Geometry: final body of the model. Coordinates: model frame, mm. A direction names the side the tool comes from. Round coordinates to 2 decimals unless told otherwise and drop trailing zeros. Loops run counter-clockwise (first coordinate to the right, second up) from the corner with the lowest first, then second, coordinate; pieces in that order, holes last. Notation, with made-up numbers: M -16.75,45.25 L 10.25,45.25 A24 cw 10.25,84.25 Z; hole C 10,21.25 d6. An arc over 180 degrees is marked long. Answer as a JSON object with one key per item and string values.
from build123d import *

# Parameters (mm, degrees)
SKETCH2_W            = 91
SKETCH2_H            = 67
BOSS_EXTRUDE10_DEPTH = 55.68
CUT_EXTRUDE13_DEPTH  = 99
CUT_EXTRUDE14_DEPTH  = 99
SKETCH28_W           = 87
SKETCH28_H           = 97.65285099
CUT_EXTRUDE16_DEPTH  = 31
SKETCH29_W           = 91
SKETCH29_H           = 35
BOSS_EXTRUDE12_DEPTH = 34.25
SKETCH30_W           = 87
SKETCH30_H           = 34.25
CUT_EXTRUDE18_DEPTH  = 32.44
SKETCH31_W           = 34.25
SKETCH31_H           = 2.550055223
BOSS_EXTRUDE13_DEPTH = 13.42
SKETCH32_W           = 34.25
SKETCH32_H           = 2.55894211
BOSS_EXTRUDE14_DEPTH = 13.42
CUT_EXTRUDE19_DEPTH  = 13.42
CUT_EXTRUDE20_DEPTH  = 13.42
SKETCH35_W           = 91
SKETCH35_H           = 35
BOSS_EXTRUDE15_DEPTH = 3
CUT_EXTRUDE21_DEPTH  = 99
SKETCH38_W           = 91
SKETCH38_H           = 34.25
BOSS_EXTRUDE16_DEPTH = 7.58
SKETCH40_W           = 87
SKETCH40_H           = 31.930310383
CUT_EXTRUDE23_DEPTH  = 7.13


with BuildPart() as part:
    # Sketch2 → Boss-Extrude10 (new body)
    with BuildSketch(Plane(origin=(0, 0, 0), x_dir=(1, 0, 0), z_dir=(0, 1, 0))):
        with Locations((45.5, 33.5)):
            Rectangle(SKETCH2_W, SKETCH2_H)
    extrude(amount=BOSS_EXTRUDE10_DEPTH)

    # Sketch24 → Cut-Extrude13 (cut)
    with BuildSketch(Plane.ZY):
        Polygon((-67, 0), (-67, 20.68), (0, 0), align=None)
    extrude(amount=-CUT_EXTRUDE13_DEPTH, mode=Mode.SUBTRACT)

    # Sketch26 → Cut-Extrude14 (cut)
    with BuildSketch(Plane.ZY):
        Polygon((0, 55.68), (0, 35), (-67, 55.68), align=None)
    extrude(amount=-CUT_EXTRUDE14_DEPTH, mode=Mode.SUBTRACT)

    # Sketch28 → Cut-Extrude16 (cut)
    with BuildSketch(Plane(origin=(0, 0, 0), x_dir=(-1, 0, 0), z_dir=(0, -0.955519618566905, -0.2949275479397551))):
        with Locations((-45.5, 48.826425495)):
            Rectangle(SKETCH28_W, SKETCH28_H)
    extrude(amount=-CUT_EXTRUDE16_DEPTH, mode=Mode.SUBTRACT)

    # Sketch29 → Boss-Extrude12 (add)
    with BuildSketch(Plane(origin=(0, 0, -67), x_dir=(-1, 0, 0), z_dir=(0, 0, -1))):
        with Locations((-45.5, 38.18)):
            Rectangle(SKETCH29_W, SKETCH29_H)
    extrude(amount=BOSS_EXTRUDE12_DEPTH)

    # Sketch30 → Cut-Extrude18 (cut)
    with BuildSketch(Plane.XZ.offset(-20.68)):
        with Locations((45.5, -84.125)):
            Rectangle(SKETCH30_W, SKETCH30_H)
    extrude(amount=-CUT_EXTRUDE18_DEPTH, mode=Mode.SUBTRACT)

    # Sketch31 → Boss-Extrude13 (add)
    with BuildSketch(Plane.ZY):
        with Locations((-84.125, 21.955027612)):
            Rectangle(SKETCH31_W, SKETCH31_H)
    extrude(amount=BOSS_EXTRUDE13_DEPTH)

    # Sketch32 → Boss-Extrude14 (add)
    with BuildSketch(Plane(origin=(91, 0, 0), x_dir=(0, 0, -1), z_dir=(1, 0, 0))):
        with Locations((84.125, 21.959471055)):
            Rectangle(SKETCH32_W, SKETCH32_H)
    extrude(amount=BOSS_EXTRUDE14_DEPTH)

    # Sketch33 → Cut-Extrude19 (cut)
    with BuildSketch(Plane(origin=(0, 23.230055223, 0), x_dir=(1, 0, 0), z_dir=(0, 1, 0))):
        Polygon((-13.42, 101.25), (0, 67), (-13.42, 67), align=None)
    extrude(amount=-CUT_EXTRUDE19_DEPTH, mode=Mode.SUBTRACT)

    # Sketch34 → Cut-Extrude20 (cut)
    with BuildSketch(Plane(origin=(0, 23.23894211, 0), x_dir=(1, 0, 0), z_dir=(0, 1, 0))):
        Polygon((91, 67), (104.42, 101.25), (104.42, 67), align=None)
    extrude(amount=-CUT_EXTRUDE20_DEPTH, mode=Mode.SUBTRACT)

    # Sketch35 → Boss-Extrude15 (add)
    with BuildSketch(Plane.XY):
        with Locations((45.5, 17.5)):
            Rectangle(SKETCH35_W, SKETCH35_H)
    extrude(amount=BOSS_EXTRUDE15_DEPTH)

    # Sketch36 → Cut-Extrude21 (cut)
    with BuildSketch(Plane.ZY):
        Polygon((0, 35), (3, 34.074029851), (3, 35), align=None)
    extrude(amount=-CUT_EXTRUDE21_DEPTH, mode=Mode.SUBTRACT)

    # Sketch38 → Boss-Extrude16 (add)
    with BuildSketch(Plane(origin=(0, 55.68, 0), x_dir=(1, 0, 0), z_dir=(0, 1, 0))):
        with Locations((45.5, 84.125)):
            Rectangle(SKETCH38_W, SKETCH38_H)
    extrude(amount=BOSS_EXTRUDE16_DEPTH)

    # Sketch40 → Cut-Extrude23 (cut)
    with BuildSketch(Plane.XZ.offset(-53.12)):
        with Locations((45.5, -85.284844808)):
            Rectangle(SKETCH40_W, SKETCH40_H)
    extrude(amount=-CUT_EXTRUDE23_DEPTH, mode=Mode.SUBTRACT)


solid = part.part
1) Section query B-B (z = -72.5). Return the cut outline in (x, y).
Results:
{"outline": "M -2.16,20.68 L 2,20.68 L 2,60.25 L 89,60.25 L 89,20.68 L 93.16,20.68 L 93.16,23.24 L 91,23.24 L 91,63.26 L 0,63.26 L 0,23.23 L -2.16,23.23 Z"}
2) Section query D-D (z = -41.5). Return the cut outline in (x, y).
Results:
{"outline": "M 0,12.81 L 2,12.81 L 2,45.25 L 89,45.25 L 89,12.81 L 91,12.81 L 91,47.81 L 0,47.81 Z"}
3) Section query C-C (y = 44). Return the cut outline in (x, z), and give its area (3 significant figures).
Results:
{"outline": "M 0,-101.25 L 2,-101.25 L 2,-37.44 L 89,-37.44 L 89,-101.25 L 91,-101.25 L 91,-29.16 L 0,-29.16 Z", "area": "1,010 mm2"}
4) Ray query, line 1 (X direction, y = 27, z = -22.5); line 2 (Z direction, x = 82, y = 21); line 3 (Z direction, x = 77, y = 60). Return the intervals inside material, ascending.
Results:
{"line 1": "0 to 2, 89 to 91", "line 2": "0 to 3", "line 3": "-69.32 to -67"}
5) Pin query (flat end, axial travel): P1, Ø4, axis at x = -6.5, z = -79, coming from the +Y side; P2, Ø3, axis at x = 13, y = 20, coming from the -Z side; P3, Ø5, axis at y = 37, z = -29, coming from the -X side. Return the tip coordinate at first contact, or that it passes through.
Results:
{"P1": "y = 23.23", "P2": "z = 0", "P3": "x = 0"}
6) Reachability of faces 4 (the flat face through (46.11, 42.93, -33.97)), 5 (the flat face through (-5, 23.23, -88)), 6 (the flat face through (-4, 20.68, -88)), 7 (the flat face through (97.62, 21.98, -83.89)), 8 (the flat face through (45, 59, -67)) from +Z, -Z, +X, -X, +Y, -Y: full face, straight path, thin tool, end or side. Return the list, or none.
Results:
{"face 4": "-Z, -Y", "face 5": "+Z, -Z, -X, +Y", "face 6": "-Z, +X, -X, -Y", "face 7": "+Z, +X, +Y, -Y", "face 8": "+Z, +X, -X, +Y"}
7) Pull-direction query (X, two-part tool) for faces 1 (the flat face through (45, 63.26, -84)), 2 (the flat face through (-6.8, 21.97, -84.36)), 3 (the flat face through (45, 16, 0)); classes: +X half, -X half, draft (parallel to the pull), parting line (faces both ways), or undercut.
Results:
{"face 1": "draft", "face 2": "-X half", "face 3": "undercut"}
